Here's how the part is built. I have some questions about the finished solid (model axes, mm). Give positions to 0.01 mm unless a question says otherwise; leave off trailing zeros. Loops run counter-clockwise (first coordinate to the right, second up) from the corner with the lowest first, then second, coordinate; pieces in that order, holes last. Notation, with made-up numbers: (60.25, -9.5) - (104.25, -9.5) arc R33 ccw to (104.25, 27.5) - close; hole circle Ø7 at (75, 63.25). An arc over 180 degrees is marked (long way). Put each result on its own line as item: value. Start each with the question number.
from build123d import *

# Parameters (mm, degrees)
F0_R     = 11.3656440934
F1_DEPTH = 25
F2_DEPTH = 32
F3_R     = 5


with BuildPart() as f1:
    # F0 (on Top) → F1 (new body)
    with BuildSketch(Plane.XY):
        with Locations((0, 23.474432528)):
            Circle(F0_R)
    extrude(amount=F1_DEPTH)

    # F2 (add): a face of the model
    f2_faces = [f1.faces().sort_by_distance(p)[0] for p in [
        (0, 23.474432528, 25),
    ]]
    extrude(f2_faces, amount=-F2_DEPTH)

    # F3
    f3_edges = [f1.edges().sort_by_distance(p)[0] for p in [
        (-11.365644, 23.474433, 25),
    ]]
    fillet(f3_edges, radius=F3_R)


solid = f1.part
1) I'm going to push flat-ended pins straight in: P1, Ø1, axis at y = 25.5, z = -3.5, coming from the -X side; P2, Ø4, axis at x = -2.5, z = 0.5, coming from the -Y side; P3, Ø5, axis at y = 26.5, z = 16.5, coming from the -X side. Where does each tip first touch, or does it pass through?
2) Suppose I cut it at A-A on z = 3. Please give me the cut outline in (x, y), plus the area to 3 significant figures.
3) I need wall thicknesses on line 1 (Z direction, x = 9.25, y = 25.75); line 2 (X direction, y = 18.25, z = 16); line 3 (Y direction, x = 6, z = 11.5). Which ranges of each line are inside material? Lowest first, please.
Ans:
1. P1: stops at x = -11.26
1. P2: stops at y = 12.12
1. P3: stops at x = -11.35
2. outline: circle Ø22.73 at (0, 23.47)
2. area: 406 mm²
3. line 1: z = -7 to 23.87
3. line 2: x = -10.09 to 10.09
3. line 3: y = 13.82 to 33.13
